Design review of the part built by this model. Coordinates are the model's own, in mm. Face numbers are marked on the shaded views. A direction names the side the tool comes from. Give positions to 0.01 mm unless a question says otherwise; leave off trailing zeros. Loops run counter-clockwise (first coordinate to the right, second up) from the corner with the lowest first, then second, coordinate; pieces in that order, holes last. Notation, with made-up numbers: (-35.5, -16.75) -> (-6.5, -16.75) arc R21 cw to (-6.5, -11.75) -> close; hole circle Ø1 at (6, -2). An arc over 180 degrees is marked (long way). Answer in a Markdown table with one row per item. Add a question column.
(1) For line 1 (Y direction, x = 5, z = 1.5); line 2 (X direction, y = 11.5, z = 6), list the stretches that pass through material, from the lowest coordinate up.
(2) For the marked faces 1, 2, 3, 4 and 5, list the 3-axis set-ups (+Z, -Z, +X, -X, +Y, -Y) from which the entire face can be reached by the end or side of a thin tool; tool diameter is ignored.
(3) Draft analysis for pull direction X (two halves, no side actions). For the marked faces 6, 7 and 8, state which applies: +X half, -X half, draft (parallel to the pull), parting line (faces both ways), or undercut.
(4) For pin 1 (3.5 mm diameter, centred on x = -2.5, z = 6.5, fed in from -Y); pin 2 (3 mm diameter, centred on x = -8, y = -5.5, fed in from -Z); pin 3 (4 mm diameter, centred on y = 9, z = 4.5, fed in from +X); pin 4 (1 mm diameter, centred on x = -5, z = 5.5, fed in from -Y), all flat-tipped, find the tip position at first contact; note any pin that passes through.
(5) Consider section B-B on x = 13. Write out the cut boundary in (y, z).
(6) Consider section A-A on z = 6. Write out the cut boundary in (x, y), then the cut area to 3 significant figures.
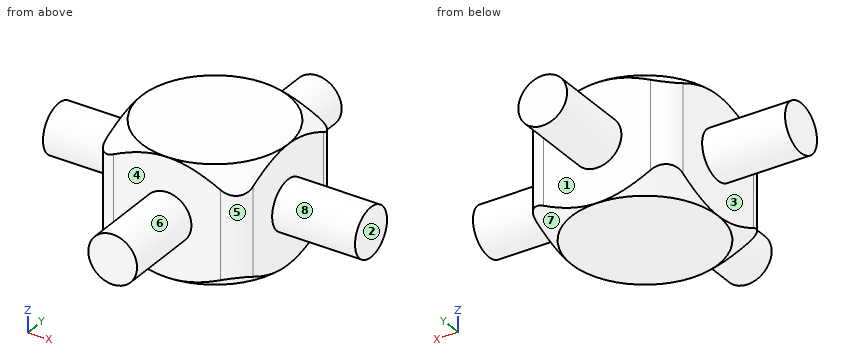
from build123d import *

# Parameters (mm, degrees)
SKETCH1_W           = 15
SKETCH1_H           = 15
BOSS_EXTRUDE1_DEPTH = 12
SKETCH2_OUTSIDE_W   = 69.544
SKETCH2_OUTSIDE_H   = 69.544
SKETCH2_OUTSIDE_R   = 7.5
CUT_EXTRUDE1_DEPTH  = 20
CUT_EXTRUDE1_DRAFT  = -50
SKETCH3_OUTSIDE_W   = 69.544
SKETCH3_OUTSIDE_H   = 69.544
SKETCH3_OUTSIDE_R   = 7.5
CUT_EXTRUDE2_DEPTH  = 20
CUT_EXTRUDE2_DRAFT  = -50
FILLET1_R           = 2
SKETCH5_R           = 2.5
BOSS_EXTRUDE2_DEPTH = 16
SKETCH6_R           = 2.5
BOSS_EXTRUDE3_DEPTH = 16


with BuildPart() as part:
    # Sketch1 → Boss-Extrude1 (new body)
    with BuildSketch(Plane.XY):
        Rectangle(SKETCH1_W, SKETCH1_H)
    extrude(amount=BOSS_EXTRUDE1_DEPTH)


with BuildPart() as cut_extrude1_tool:
    # Sketch2 outside → Cut-Extrude1 (with draft: the straight prism first)
    with BuildSketch(Plane.XY.offset(12)):
        Rectangle(SKETCH2_OUTSIDE_W, SKETCH2_OUTSIDE_H)
        Circle(SKETCH2_OUTSIDE_R, mode=Mode.SUBTRACT)
    extrude(amount=-CUT_EXTRUDE1_DEPTH)
    # Cut-Extrude1: the draft: its side faces are tilted about the plane it starts from
    cut_extrude1_sides = [cut_extrude1_tool.faces().sort_by_distance(p)[0] for p in [
        (0, -34.772, 2),
        (34.772, 0, 2),
        (0, 34.772, 2),
        (-34.772, 0, 2),
        (-7.5, 0, 2),
    ]]
    draft(cut_extrude1_sides, Plane.XY.offset(12), CUT_EXTRUDE1_DRAFT)


with BuildPart() as part_1:
    add(part.part)

    # Cut-Extrude1: cut by cut_extrude1_tool
    add(cut_extrude1_tool.part, mode=Mode.SUBTRACT)


with BuildPart() as cut_extrude2_tool:
    # Sketch3 outside → Cut-Extrude2 (with draft: the straight prism first)
    with BuildSketch(Plane(origin=(0, 0, 0), x_dir=(-1, 0, 0), z_dir=(0, 0, -1))):
        Rectangle(SKETCH3_OUTSIDE_W, SKETCH3_OUTSIDE_H)
        Circle(SKETCH3_OUTSIDE_R, mode=Mode.SUBTRACT)
    extrude(amount=-CUT_EXTRUDE2_DEPTH)
    # Cut-Extrude2: the draft: its side faces are tilted about the plane it starts from
    cut_extrude2_sides = [cut_extrude2_tool.faces().sort_by_distance(p)[0] for p in [
        (0, -34.772, 10),
        (-34.772, 0, 10),
        (0, 34.772, 10),
        (34.772, 0, 10),
        (7.5, 0, 10),
    ]]
    draft(cut_extrude2_sides, Plane(origin=(0, 0, 0), x_dir=(-1, 0, 0), z_dir=(0, 0, -1)), CUT_EXTRUDE2_DRAFT)


with BuildPart() as part_2:
    add(part_1.part)

    # Cut-Extrude2: cut by cut_extrude2_tool
    add(cut_extrude2_tool.part, mode=Mode.SUBTRACT)

    # Fillet1
    fillet1_edges = [part_2.edges().sort_by_distance(p)[0] for p in [
        (7.5, -7.5, 6),
        (7.5, 7.5, 6),
        (-7.5, 7.5, 6),
        (-7.5, -7.5, 6),
    ]]
    fillet(fillet1_edges, radius=FILLET1_R)

    # Sketch5 → Boss-Extrude2 (add, symmetric)
    with BuildSketch(Plane(origin=(0, 0, 0), x_dir=(1, 0, 0), z_dir=(0, 1, 0))):
        with Locations(Location((0, -6, 0), (0, 0, 270))):
            Circle(SKETCH5_R)
    extrude(amount=BOSS_EXTRUDE2_DEPTH, both=True)

    # Sketch6 → Boss-Extrude3 (add, symmetric)
    with BuildSketch(Plane(origin=(0, 0, 0), x_dir=(0, 0, -1), z_dir=(1, 0, 0))):
        with Locations((-6, 0)):
            Circle(SKETCH6_R)
    extrude(amount=BOSS_EXTRUDE3_DEPTH, both=True)


solid = part_2.part
Values follow:
| question | item | result |
|---|---|---|
| 1 | line 1 | -7.5 to 7.5 |
| 1 | line 2 | -2.5 to 2.5 |
| 2 | face 1 | +Y |
| 2 | face 2 | +Z, -Z, +X, +Y, -Y |
| 2 | face 3 | -X |
| 2 | face 4 | -Y |
| 2 | face 5 | +Z, -Z, +X, -Y |
| 3 | face 6 | parting line |
| 3 | face 7 | +X half |
| 3 | face 8 | draft |
| 4 | pin 1 | y = -16 |
| 4 | pin 2 | z = 0.59 |
| 4 | pin 3 | x = 6.82 |
| 4 | pin 4 | y = -7.5 |
| 5 | outline | circle Ø5 at (0, 6) |
| 6 | outline | (-16, -2.5) -> (-7.5, -2.5) -> (-7.5, -5.5) arc R2 ccw to (-5.5, -7.5) -> (-2.5, -7.5) -> (-2.5, -16) -> (2.5, -16) -> (2.5, -7.5) -> (5.5, -7.5) arc R2 ccw to (7.5, -5.5) -> (7.5, -2.5) -> (16, -2.5) -> (16, 2.5) -> (7.5, 2.5) -> (7.5, 5.5) arc R2 ccw to (5.5, 7.5) -> (2.5, 7.5) -> (2.5, 16) -> (-2.5, 16) -> (-2.5, 7.5) -> (-5.5, 7.5) arc R2 ccw to (-7.5, 5.5) -> (-7.5, 2.5) -> (-16, 2.5) -> close |
| 6 | area | 392 mm2 |
